Autodesk Inventor part; units mm, degrees
ref_plane "YZ Plane" through (0, 0, 0) normal (1, 0, 0) x (0, 1, 0)
ref_plane "XZ Plane" through (0, 0, 0) normal (0, 1, 0) x (-1, 0, 0)
ref_plane "XY Plane" through (0, 0, 0) normal (0, 0, 1) x (1, 0, 0)
sketch "草图1" plane through (0, 0, 0) normal (0, 1, 0) x (-1, 0, 0)
  line L0 (35.3553, 35.3553) -> (-35.3553, 35.3553)
  line L1 (-35.3553, 35.3553) -> (-35.3553, -35.3553)
  line L2 (-35.3553, -35.3553) -> (35.3553, -35.3553)
  line L3 (35.3553, -35.3553) -> (35.3553, 35.3553)
  line L4 (35.3553, 35.3553) -> (-35.3553, -35.3553)
  line L5 (35.3553, -35.3553) -> (-35.3553, 35.3553)
  line L6 (-22.981, 47.7297) -> (-47.7297, 22.981)
  line L7 (-47.7297, -22.981) -> (-22.981, -47.7297)
  line L8 (22.981, -47.7297) -> (47.7297, -22.981)
  line L9 (47.7297, 22.981) -> (22.981, 47.7297)
  line L10 (22.981, 47.7297) -> (-22.981, 47.7297)
  line L11 (47.7297, 22.981) -> (47.7297, -22.981)
  line L12 (22.981, -47.7297) -> (-22.981, -47.7297)
  line L13 (-47.7297, -22.981) -> (-47.7297, 22.981)
  circle A0 centre (41.0122, 25.4558) radius 1.65
  circle A1 centre (25.4558, 41.0122) radius 1.65
  circle A2 centre (-41.0122, 25.4558) radius 1.65
  circle A3 centre (-25.4558, 41.0122) radius 1.65
  circle A4 centre (-25.4558, -41.0122) radius 1.65
  circle A5 centre (-41.0122, -25.4558) radius 1.65
  circle A6 centre (41.0122, -25.4558) radius 1.65
  circle A7 centre (25.4558, -41.0122) radius 1.65
  line L14 (-47.7297, -22.981) -> (-77.7297, -22.981)
  line L15 (-77.7297, -22.981) -> (-77.7297, 22.981)
  line L16 (-47.7297, 22.6987) -> (-47.7297, -22.981)
  line L17 (-47.7297, 22.981) -> (-77.7297, 22.981)
  line L18 (47.7297, -22.981) -> (77.7297, -22.981)
  line L19 (77.7297, -22.981) -> (77.7297, 22.981)
  line L20 (77.7297, 22.981) -> (47.7297, 22.981)
  point P0 (0, 0)
  point P1 (0, 0)
  point P2 (0, 0)
  point P3 (-35.3553, -35.3553)
  point P4 (35.3553, -35.3553)
  point P5 (35.3553, 35.3553)
  point P6 (0, 0)
  dimension "d4" = 100
  dimension "d5" = 35
  dimension "d6" = 45
  dimension "d7" = 360
  dimension "d8" = 3.3
  dimension "d9" = 3
  dimension "d10" = 11
  dimension "d18" = 360
  dimension "d20" = 30
  dimension "d23" = 30
extrude "拉伸1" add sketch "草图1" along normal blind 3
properties part number "下板"
Model file for the job. Use its own axes, mm. A direction names the side the tool comes from. Give positions to 0.01 mm unless a question says otherwise; leave off trailing zeros. Loops run counter-clockwise (first coordinate to the right, second up) from the corner with the lowest first, then second, coordinate; pieces in that order, holes last. Notation, with made-up numbers: (4.5, 45.5) - (17.5, 45.5) arc R5 ccw to (17.5, 54.5) - close; hole circle Ø8 at (-11, -19.75). An arc over 180 degrees is marked (long way). Use one line per item in the form item = value.
(1) Drill centre lines: L1, parallel to Z at x = 41.5, y = 1.6; L2, parallel to Z at x = 25, y = 2; L3, parallel to X at y = 1.35, z = 24. Where is each one in solid material? Low to high.
Determined:
L1 = -29.21 to -27.03, -23.88 to 23.88, 27.03 to 29.21
L2 = -45.71 to -42.6, -39.43 to 39.43, 42.6 to 45.71
L3 = -46.71 to -41.79, -40.24 to 40.24, 41.79 to 46.71
(2) Cut at A-A (y = 0.9). Count the separate pieces of the cut face and the enclosed holes in it, then the cut area to 3 significant figures.
Determined:
separate_pieces = 1
enclosed_holes = 8
area = 10,600 mm^2
(3) Cut at C-C (z = -30.5). Give the cut face in (x, y), then the cut area to 3 significant figures.
Determined:
outline = (-40.21, 0) - (40.21, 0) - (40.21, 3) - (-40.21, 3) - close
area = 241 mm^2
(4) 3-axis set-ups, long thin cutter, end or side, ignore diameter. For faces 5 (the face through (77.73, 1, 0)), 6 (the face through (0, 1, 47.73)), 7 (the face through (-63, 1, 22.981)), 8 (the face through (63, 1, 22.981)), 9 (the face through (-63, 1, -22.981)): which of +Z, -Z, +X, -X, +Y, -Y reach the whole face in a straight line?
Determined:
face_5 = +Z, -Z, +X, +Y, -Y
face_6 = +Z, +X, -X, +Y, -Y
face_7 = +Z, -X, +Y, -Y
face_8 = +Z, +X, +Y, -Y
face_9 = -Z, -X, +Y, -Y
(5) Cut at B-B (x = 57). Give the cut face in (y, z), then the cut area to 3 significant figures.
Determined:
outline = (0, -22.98) - (3, -22.98) - (3, 22.98) - (0, 22.98) - close
area = 138 mm^2
(6) Drop a flat-ended pin along its axis: P1, Ø1.5, axis at x = 67, y = 1.5, coming from the +Z side. Give the stop position or say it passes through.
Determined:
P1 = 22.98
(7) Pull direction X, two halves, no side cores. Call faces 1 (the face through (42.66, 1.48, -25.53)), 2 (the face through (26.672, 1.479, 39.897)), 3 (the face through (63, 1, -22.981)), 4 (the face through (-77.73, 1, 0)): pulls with the +X half, pulls with the -X half, needs draft (parallel to the pull), parting line crosses it, or undercut.
Determined:
face_1 = undercut
face_2 = undercut
face_3 = needs draft
face_4 = pulls with the -X half
